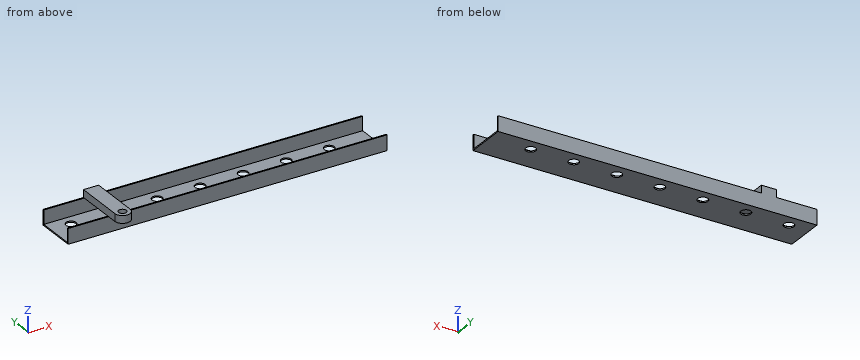
```python
from build123d import *

# Parameters (mm, degrees)
BASE_EXTRUDE_THIN_DEPTH = 800.1
SKETCH2_R               = 12.7
CUT_EXTRUDE1_DEPTH      = 808.424411323
LPATTERN1_COUNT         = 7
LPATTERN1_PITCH         = 107.95
BOSS_EXTRUDE1_START     = 38.1
BOSS_EXTRUDE1_OUTLINE_R = 9.525
BOSS_EXTRUDE1_DEPTH     = 19.05


# Read off the part's stored shape, not the designer's step: Boss-Extrude1
with BuildPart() as part:
    # Sketch1 → Base-Extrude-Thin (new body)
    with BuildSketch(Plane(origin=(0, 0, 0), x_dir=(0, 0, -1), z_dir=(1, 0, 0))):
        Polygon((-38.1, 0), (0, 0), (0, -101.6), (-38.1, -101.6), (-38.1, -98.425), (-3.175, -98.425), (-3.175, -3.175), (-38.1, -3.175), align=None)
    extrude(amount=BASE_EXTRUDE_THIN_DEPTH)

    # Sketch2 → Cut-Extrude1 (cut, through all)
    with BuildSketch(Plane(origin=(0, 0, 0), x_dir=(-1, 0, 0), z_dir=(0, 0, -1))):
        with Locations(Location((-50.8, -31.75, 0), (0, 0, 90))):
            Circle(SKETCH2_R)
    cut_extrude1 = extrude(amount=-CUT_EXTRUDE1_DEPTH, mode=Mode.SUBTRACT)

    # LPattern1: Cut-Extrude1 ×7
    with Locations(*[(i * LPATTERN1_PITCH, 0, 0) for i in range(1, LPATTERN1_COUNT)]):
        add(cut_extrude1, mode=Mode.SUBTRACT)

    # Boss-Extrude1 outline → Boss-Extrude1 (add)
    with BuildSketch(Plane.XY.offset(BOSS_EXTRUDE1_START)):
        with BuildLine():
            Line((101.6, 0), (101.6, -127))
            ThreePointArc((101.6, -127), (120.65, -146.05), (139.7, -127))
            Line((139.7, -127), (139.7, 0))
            Line((139.7, 0), (101.6, 0))
        make_face()
        with Locations((120.65, -127)):
            Circle(BOSS_EXTRUDE1_OUTLINE_R, mode=Mode.SUBTRACT)
    extrude(amount=BOSS_EXTRUDE1_DEPTH)


solid = part.part
```
Source: CAD feature listing. Evaluate the final solid. Frame: model axes, mm. Round coordinates to 2 decimals unless told otherwise and drop trailing zeros. Loops run counter-clockwise (first coordinate to the right, second up) from the corner with the lowest first, then second, coordinate; pieces in that order, holes last. Notation, with made-up numbers: M 22,66.25 L 52,66.25 A12 ccw 52,72.25 Z; hole C 31,11.5 d4. An arc over 180 degrees is marked long. Put each result on its own line as item: value.
(1) Section C-C, the plane y = -51. Return loops of the section in (x, z) (3 decimals), and give its area (3 significant figures).
Solutions:
outline: M 0,0 L 800.1,0 L 800.1,3.175 L 0,3.175 Z; M 101.6,38.1 L 139.7,38.1 L 139.7,57.15 L 101.6,57.15 Z
area: 3,270 mm²
(2) Section B-B, the plane x = 158.75. Return loops of the section in (y, z) (3 decimals).
Solutions:
outline: M -101.6,0 L -44.45,0 L -44.45,3.175 L -98.425,3.175 L -98.425,38.1 L -101.6,38.1 Z; M -19.05,0 L 0,0 L 0,38.1 L -3.175,38.1 L -3.175,3.175 L -19.05,3.175 Z
(3) Section A-A, the plane z = 12.5. Return loops of the section in (x, y) (3 decimals), and give its area (3 significant figures).
Solutions:
outline: M 0,-101.6 L 800.1,-101.6 L 800.1,-98.425 L 0,-98.425 Z; M 0,-3.175 L 800.1,-3.175 L 800.1,0 L 0,0 Z
area: 5,080 mm²
(4) First-contact query: pin 1 (17.5 mm diameter, centred on x = 233.5, z = 19.5, fed in from -Y); pin 2 (10 mm diameter, centred on y = -81.5, z = 44, fed in from +X); pin 3 (15 mm diameter, centred on y = -63.5, z = 43.5, fed in from -X); pin 4 (4 mm diameter, centred on x = 424, z = 24, fed in from +Y). Flat tips, straight axial feed; report the tip coordinate or a pass-through.
Solutions:
pin 1: y = -101.6
pin 2: x = 139.7
pin 3: x = 101.6
pin 4: y = 0
(5) Ray query, line 1 (Y direction, x = 198.5, z = 29.5) (3 decimals); line 2 (Z direction, x = 136, y = -44) (3 decimals); line 3 (Y direction, x = 482, z = 2). Return the intervals inside material, ascending. Write a range as [from, to].
Solutions:
line 1: [-101.6, -98.425], [-3.175, 0]
line 2: [0, 3.175], [38.1, 57.15]
line 3: [-101.6, -44.44], [-19.06, 0]
(6) Section D-D, the plane z = 45. Return loops of the section in (x, y) (3 decimals).
Solutions:
outline: M 101.6,-127 A19.05 ccw 139.7,-127 L 139.7,0 L 101.6,0 Z; hole C 120.65,-127 d19.05
